Source: CAD feature listing. Evaluate the final solid. Frame: model axes, mm. A direction names the side the tool comes from. Round coordinates to 2 decimals unless told otherwise and drop trailing zeros. Order: outer loops, then holes, each group sorted by start corner. A loop starts at its lowest first (then second) coordinate and runs counter-clockwise, first axis right, second up. Notation, with made-up numbers: (32.25, 64.5) -> (46.25, 64.5) arc R24 ccw to (46.25, 96.5) -> close; hole circle Ø3 at (23.5, 11). An arc over 180 degrees is marked (long way). Answer as CSV lines item,"result". Start each with the question number.
(1) Contact query for flat-ended pins moving along their axis: P1, Ø1.8, axis at x = -0.5, z = 0, coming from the +Y side; P2, Ø2, axis at y = -2.5, z = -1.5, coming from the +X side; P3, Ø0.6, axis at x = 0.5, y = 5.5, coming from the -Z side. Output: stop coordinate, or through.
(2) Set-up query: faces 4 (the flat face through (-1.39, 4.78, 0.79)), 5 (the cylindrical face through (-0.03, -0.45, 2.87)). Return all of +Z, -Z, +X, -X, +Y, -Y with unobstructed straight access to the full face (end or side cutting, diameter ignored); none if empty.
(3) Line query: line 1 along X through (y, z) = (-2.75, -0.75); line 2 along Z through (x, y) = (3.25, -3); line 3 along X through (y, z) = (-2, 3). Output: solid intervals per line, ascending. Write a range as from..to.
(4) Pull-direction query (Z, two-part tool) for faces 1 (the cylindrical face through (-2.5, -0.45, 1.41)), 2 (the cylindrical face through (3.233, 4.499, -1.341)), 3 (the flat face through (0, 7, 2)); classes: +Z half, -Z half, draft (parallel to the pull), parting line (faces both ways), or undercut.
(5) Section query B-B (y = 4.75). Output: boundary loops of the cut face in (x, z).
(6) Section query A-A (y = -2). Output: boundary loops of the cut face in (x, z), plus the area to 3 significant figures.
```python
from build123d import *

# Parameters (mm, degrees)
F3_DEPTH = 5
F5_R     = 1.5
F6_DEPTH = 7
F7_R     = 1.5
F8_R     = 0.5


with BuildPart() as f1:
    # F0 (on Top) → F1 (revolve)
    with BuildSketch(Plane.XY):
        Polygon((3.5, 1), (3.5, 7), (0, 7), (0, -7), (5.5, -7), (5.5, 0), align=None)
    revolve(axis=Axis((0, -5.739396, 0), (0, -1, 0)))

    # F2 (on face) → F3 (cut)
    with BuildSketch(Plane(origin=(0, 7, 0), x_dir=(-1, 0, 0), z_dir=(0, 1, 0))):
        Polygon((0.92376, -1.6), (1.847521, 0), (0.92376, 1.6), (-0.92376, 1.6), (-1.847521, 0), (-0.92376, -1.6), align=None)
    extrude(amount=-F3_DEPTH, mode=Mode.SUBTRACT)

    # F5
    f5_edges = [f1.edges().sort_by_distance(p)[0] for p in [
        (-5.5, 0, 0),
        (-3.5, 1, 0),
    ]]
    fillet(f5_edges, radius=F5_R)

    # F4 (on face) → F6 (cut)
    with BuildSketch(Plane.XZ.offset(7)):
        Polygon((1.905256, -3.3), (3.810512, 0), (1.905256, 3.3), (-1.905256, 3.3), (-3.810512, 0), (-1.905256, -3.3), align=None)
    extrude(amount=-F6_DEPTH, mode=Mode.SUBTRACT)

    # F7
    f7_edges = [f1.edges().sort_by_distance(p)[0] for p in [
        (0, 0, -3.3),
        (2.857884, 0, -1.65),
        (2.857884, 0, 1.65),
        (0, 0, 3.3),
        (-2.857884, 0, 1.65),
        (-2.857884, 0, -1.65),
    ]]
    fillet(f7_edges, radius=F7_R)

    # F8
    f8_edges = [f1.edges().sort_by_distance(p)[0] for p in [
        (0, 2, -1.6),
        (-1.385641, 2, -0.8),
        (1.385641, 2, -0.8),
        (-1.385641, 2, 0.8),
        (0, 2, 1.6),
        (1.385641, 2, 0.8),
    ]]
    fillet(f8_edges, radius=F8_R)


solid = f1.part
```
Answer block:
1,P1,"y = 2.06"
1,P2,"x = 5.48"
1,P3,"z = -3.49"
2,face 4,"+Y"
2,face 5,"-Y"
3,line 1,"-5.45..-3.38, 3.38..5.45"
3,line 2,"-4.44..-0.97, 0.97..4.44"
3,line 3,"-4.61..-2.08, 2.08..4.61"
4,face 1,"undercut"
4,face 2,"parting line"
4,face 3,"draft"
5,outline,"circle Ø7 at (0, 0); hole (-1.85, 0) -> (-0.92, -1.6) -> (0.92, -1.6) -> (1.85, 0) -> (0.92, 1.6) -> (-0.92, 1.6) -> close"
6,outline,"circle Ø11 at (0, 0); hole (-3.81, 0) -> (-1.91, -3.3) -> (1.91, -3.3) -> (3.81, 0) -> (1.91, 3.3) -> (-1.91, 3.3) -> close"
6,area,"57.3 mm2"
